The listing builds one solid part. Answer for the finished solid, in the listing's coordinates (mm). A direction names the side the tool comes from. Give positions to 0.01 mm unless a question says otherwise; leave off trailing zeros. Write each loop counter-clockwise with the first axis right and the second up, starting at its lowest first coordinate (ties: lowest second). Pieces come first, ordered by that corner, then holes. Notation, with made-up numbers: (72.5, -19) -> (116.5, -19) arc R22 ccw to (116.5, -11) -> close; hole circle Ø10 at (-37, 62). An arc over 180 degrees is marked (long way). Put each result on its own line as item: value. Start each with the question number.
1) A cutting plane is placed at A-A (x = -25). Write down the section's boundary in (y, z), then the cut area to 3 significant figures.
2) For a pull along X with two mould halves and no side action, classify faces 4 (the cylindrical face through (-3.282, -40.399, 3.944)), 5 (the flat face through (5.9, 49.6, 5.9)), 6 (the flat face through (-0.314, 50.155, 9.972)), 7 (the flat face through (29, -75, 15)) as released by +X, released by -X, zero draft, split by the parting line, or undercut.
3) Find the intervals of material crossed by line 1 along Z through (x, y) = (-21.5, 26); line 2 along Z through (x, y) = (10.5, 28); line 3 along X through (y, z) = (-45, 2.25), in increasing order. Write a range as from..to.
4) A cutting plane is placed at D-D (y = 6). Write down the section's boundary in (x, z).
5) A cutting plane is placed at C-C (y = -52). Write down the section's boundary in (x, z), then the cut area to 3 significant figures.
6) A cutting plane is placed at B-B (z = 3.75). Write down the section's boundary in (x, y).
7) For faces 1 (the cylindrical face through (9.658, -5.813, 3.944)), 2 (the flat face through (-22.185, -21.114, 4.583)), 3 (the flat face through (-16.07, -35.91, 9.97)), determine the directions among +Z, -Z, +X, -X, +Y, -Y from which every point of the face is accessible in a straight line to the end or side of a thin tool.
8) Flat-ended cylindrical pins translate along their axes: pin 1 Ø10 at (x, y) = (-22.5, -19.5) entering from +Z; pin 2 Ø1.5 at (y, z) = (-44.5, 11.5) entering from -X; pin 3 Ø8 at (x, z) = (6, 7) entering from -Y; pin 4 Ø5 at (x, y) = (27.21, -70.71) entering from -Z. Find the tip coordinate at first contact, or state that the pin passes through.
from build123d import *

# Parameters (mm, degrees)
SKETCH1_R           = 3
SKETCH1_R_2         = 4.25
BOSS_EXTRUDE1_DEPTH = 8
SKETCH2_R           = 4.25
BOSS_EXTRUDE2_DEPTH = 4
SKETCH3_R           = 6.5
SKETCH3_R_2         = 4.25
BOSS_EXTRUDE3_DEPTH = 3


with BuildPart() as part:
    # Sketch1 → Boss-Extrude1 (new body)
    with BuildSketch(Plane.XY):
        with BuildLine():
            Line((-15.213203436, 14.142135624), (-15.171572875, 14.183766184))
            ThreePointArc((-15.171572875, 14.183766184), (-11.231737479, 14.96744817), (-9, 11.627416998))
            Line((-9, 11.627416998), (-9, -11.627416998))
            ThreePointArc((-9, -11.627416998), (-11.231737479, -14.96744817), (-15.171572875, -14.183766184))
            Line((-15.171572875, -14.183766184), (-15.213203436, -14.142135624))
            Line((-15.213203436, -14.142135624), (-29.355339059, -28.284271247))
            Line((-29.355339059, -28.284271247), (20.142135624, -77.781745931))
            ThreePointArc((20.142135624, -77.781745931), (31.996800536, -79.492317987), (36.988958333, -68.60482528))
            Line((36.988958333, -68.60482528), (13.071067812, 42.426406871))
            Line((13.071067812, 42.426406871), (-1.071067812, 56.568542495))
            Line((-1.071067812, 56.568542495), (-29.355339059, 28.284271247))
            Line((-29.355339059, 28.284271247), (-15.213203436, 14.142135624))
        make_face()
        with Locations((-1.071067812, 42.426406871)):
            Circle(SKETCH1_R, mode=Mode.SUBTRACT)
        with Locations((-15.213203436, 28.284271247)):
            Circle(SKETCH1_R, mode=Mode.SUBTRACT)
        with Locations((-15.213203436, -28.284271247)):
            Circle(SKETCH1_R, mode=Mode.SUBTRACT)
        with Locations((-1.071067812, -42.426406871)):
            Circle(SKETCH1_R, mode=Mode.SUBTRACT)
        with Locations((27.213203436, -70.710678119)):
            Circle(SKETCH1_R_2, mode=Mode.SUBTRACT)
        with BuildLine():
            Line((6, -9.798512067), (6, -33.69848481))
            ThreePointArc((6, -33.69848481), (6.30448187, -35.229218539), (7.171572875, -36.526911935))
            Line((7.171572875, -36.526911935), (13.733563505, -43.088902565))
            ThreePointArc((13.733563505, -43.088902565), (18.47542947, -43.773131388), (20.472292589, -39.418134305))
            Line((20.472292589, -39.418134305), (13.910301959, -8.956170931))
            ThreePointArc((13.910301959, -8.956170931), (9.576448254, -5.820999789), (6, -9.798512067))
        make_face(mode=Mode.SUBTRACT)
    extrude(amount=BOSS_EXTRUDE1_DEPTH)

    # Sketch2 → Boss-Extrude2 (add)
    with BuildSketch(Plane.XY.offset(8)):
        with BuildLine():
            Line((24.355165698, -57.443143037), (3.641635622, 38.712860541))
            ThreePointArc((3.641635622, 38.712860541), (4.918487685, 42.780278254), (3.171572875, 46.669047558))
            Line((3.171572875, 46.669047558), (-3.899494937, 53.74011537))
            Line((-3.899494937, 53.74011537), (-1.071067812, 56.568542495))
            Line((-1.071067812, 56.568542495), (13.071067812, 42.426406871))
            Line((13.071067812, 42.426406871), (36.988958333, -68.60482528))
            ThreePointArc((36.988958333, -68.60482528), (31.996800536, -79.492317987), (20.142135624, -77.781745931))
            Line((20.142135624, -77.781745931), (-29.355339059, -28.284271247))
            Line((-29.355339059, -28.284271247), (-26.526911935, -25.455844123))
            Line((-26.526911935, -25.455844123), (-5.313708499, -46.669047558))
            ThreePointArc((-5.313708499, -46.669047558), (-1.071067812, -48.426406871), (3.171572875, -46.669047558))
            Line((3.171572875, -46.669047558), (17.616436614, -61.113911297))
            ThreePointArc((17.616436614, -61.113911297), (22.358302578, -61.79814012), (24.355165698, -57.443143037))
        make_face()
        with Locations((27.213203436, -70.710678119)):
            Circle(SKETCH2_R, mode=Mode.SUBTRACT)
    extrude(amount=BOSS_EXTRUDE2_DEPTH)

    # Sketch3 → Boss-Extrude3 (add)
    with BuildSketch(Plane.XY.offset(12)):
        with Locations((27.213203436, -70.710678119)):
            Circle(SKETCH3_R)
        with Locations((27.213203436, -70.710678119)):
            Circle(SKETCH3_R_2, mode=Mode.SUBTRACT)
    extrude(amount=BOSS_EXTRUDE3_DEPTH)


solid = part.part
Reply:
1. outline: (-32.64, 0) -> (-23.93, 0) -> (-23.93, 8) -> (-26.98, 8) -> (-26.98, 12) -> (-32.64, 12) -> close; (23.93, 0) -> (32.64, 0) -> (32.64, 8) -> (23.93, 8) -> close
1. area: 162 mm2
2. face 4: undercut
2. face 5: released by +X
2. face 6: released by -X
2. face 7: zero draft
3. line 1: z = 0..8
3. line 2: z = 0..12
3. line 3: x = -12.64..-2.61, 0.47..31.9
4. outline: (-9, 0) -> (20.92, 0) -> (20.92, 12) -> (10.69, 12) -> (10.69, 8) -> (-9, 8) -> close
5. outline: (-5.64, 0) -> (33.41, 0) -> (33.41, 12) -> (23.18, 12) -> (23.18, 8) -> (8.5, 8) -> (8.5, 12) -> (-5.64, 12) -> close
5. area: 410 mm2
6. outline: (-29.36, -28.28) -> (20.14, -77.78) arc R10 ccw to (36.99, -68.6) -> (13.07, 42.43) -> (-1.07, 56.57) -> (-29.36, 28.28) -> (-15.21, 14.14) -> (-15.17, 14.18) arc R3.62 cw to (-9, 11.63) -> (-9, -11.63) arc R3.62 cw to (-15.17, -14.18) -> (-15.21, -14.14) -> close; hole circle Ø6 at (-15.21, -28.28); hole circle Ø6 at (-15.21, 28.28); hole circle Ø6 at (-1.07, -42.43); hole circle Ø6 at (-1.07, 42.43); hole (6, -33.7) arc R4 ccw to (7.17, -36.53) -> (13.73, -43.09) arc R4 ccw to (20.47, -39.42) -> (13.91, -8.96) arc R4 ccw to (6, -9.8) -> close; hole circle Ø8.5 at (27.21, -70.71)
7. face 1: +Z, -Z
7. face 2: +Z, -Z, -X
7. face 3: +Z, +Y
8. pin 1: stops at z = 8
8. pin 2: stops at x = -13.89
8. pin 3: stops at y = -67.64
8. pin 4: passes through
